Geometry check sheet. Reference: drawing and pictorial views, mm from the part's lowest x, y, z. A direction names the side the tool comes from. Give positions to 0.01 mm unless a question says otherwise; leave off trailing zeros. Write each loop counter-clockwise with the first axis right and the second up, starting at its lowest first coordinate (ties: lowest second). Pieces come first, ordered by that corner, then holes. Notation, with made-up numbers: (-5.5, 31.25) - (49.5, 31.25) arc R22 ccw to (49.5, 54.25) - close; hole circle Ø4 at (67, 53). An arc over 180 degrees is marked (long way). Write item = value, one per line. Start each with the question number.
(1) Section check A-A, the plane x = 57. Enter the section's corners in (y, z).
(2) Section check C-C, the plane z = 22. Enter the section's corners in (x, y), plus the area to 3 significant figures.
(3) Section check D-D, the plane x = 50. Enter the section's corners in (y, z).
(4) Section check B-B, the plane y = 22. Enter the section's corners in (x, z), plus the area to 3 significant figures.
(5) Draft check along X on the marked faces 1, 2 and 3. Enter one of: pulls with the +X half, pulls with the -X half, needs draft (parallel to the pull), parting line crosses it, or undercut.
(6) Depth check by flat-ended pin: pin 1 Ø4 at (x, y) = (13, 38) entering from -Z; pin 2 Ø0.9 at (y, z) = (22, 43) entering from +X; pin 3 Ø12 at (x, y) = (52, 25) entering from -Z. Enter the tip coordinate at first touch or a pass-through.
(7) Access from +Z, -Z, +X, -X, +Y, -Y to the whole of each face (thin tool, end or side, straight path). Record for the marked faces 4, 5, 6, 7 and 8.
(8) Thickness scan on L1, parallel to Y at x = 56.5, z = 10.5 (1 decimal); L2, parallel to Y at x = 57, z = 10; L3, parallel to X at y = 27.5, z = 22. Record the ranges inside material, lowest first.
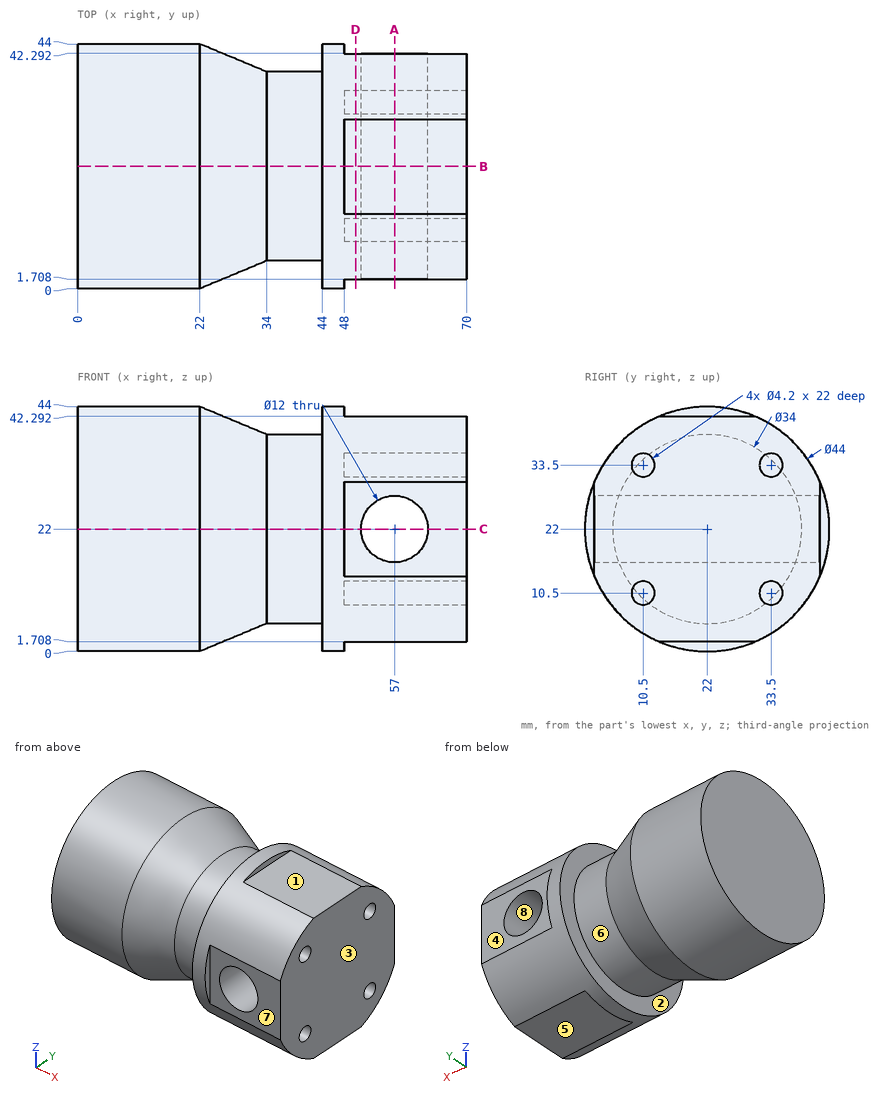
Model answer:
q1.outline = (1.71, 13.5) arc R22 ccw to (13.5, 1.71) - (30.5, 1.71) arc R22 ccw to (42.29, 13.5) - (42.29, 16) - (1.71, 16) - close; (1.71, 28) - (42.29, 28) - (42.29, 30.5) arc R22 ccw to (30.5, 42.29) - (13.5, 42.29) arc R22 ccw to (1.71, 30.5) - close; hole circle Ø4.2 at (10.5, 10.5); hole circle Ø4.2 at (10.5, 33.5); hole circle Ø4.2 at (33.5, 10.5); hole circle Ø4.2 at (33.5, 33.5)
q2.outline = (0, 0) - (22, 0) - (34, 5) - (44, 5) - (44, 0) - (48, 0) - (48, 1.71) - (51, 1.71) - (51, 42.29) - (48, 42.29) - (48, 44) - (44, 44) - (44, 39) - (34, 39) - (22, 44) - (0, 44) - close; (63, 1.71) - (70, 1.71) - (70, 42.29) - (63, 42.29) - close
q2.area = 2,360 mm²
q3.outline = (1.71, 13.5) arc R22 ccw to (13.5, 1.71) - (30.5, 1.71) arc R22 ccw to (42.29, 13.5) - (42.29, 30.5) arc R22 ccw to (30.5, 42.29) - (13.5, 42.29) arc R22 ccw to (1.71, 30.5) - close; hole circle Ø4.2 at (10.5, 10.5); hole circle Ø4.2 at (10.5, 33.5); hole circle Ø4.2 at (33.5, 10.5); hole circle Ø4.2 at (33.5, 33.5)
q4.outline = (0, 0) - (22, 0) - (34, 5) - (44, 5) - (44, 0) - (48, 0) - (48, 1.71) - (70, 1.71) - (70, 42.29) - (48, 42.29) - (48, 44) - (44, 44) - (44, 39) - (34, 39) - (22, 44) - (0, 44) - close; hole circle Ø12 at (57, 22)
q4.area = 2,730 mm²
q5.face_1 = needs draft
q5.face_2 = undercut
q5.face_3 = pulls with the +X half
q6.pin_1 = 5.03
q6.pin_2 = 48
q6.pin_3 = 0
q7.face_4 = +Z, -Z, +X, +Y
q7.face_5 = -Z, +X, +Y, -Y
q7.face_6 = none
q7.face_7 = +Z, -Z, +X, -Y
q7.face_8 = +Y, -Y
q8.L1 = 3.2 to 8.4, 12.6 to 31.4, 35.6 to 40.8
q8.L2 = 3.56 to 8.46, 12.54 to 31.46, 35.54 to 40.44
q8.L3 = 0 to 51, 63 to 70
